Here's the drawing with two shaded views (mm, measured from the low corner). I have some questions. Give positions to 0.01 mm unless a question says otherwise; leave off trailing zeros. Order: outer loops, then holes, each group sorted by start corner. A loop starts at its lowest first (then second) coordinate and runs counter-clockwise, first axis right, second up. Notation, with made-up numbers: M 42.5,13 L 59.5,13 A6 cw 59.5,21 Z; hole C 7.5,87 d4. An arc over 180 degrees is marked long. Use a Markdown table: item, result. Add a question column.
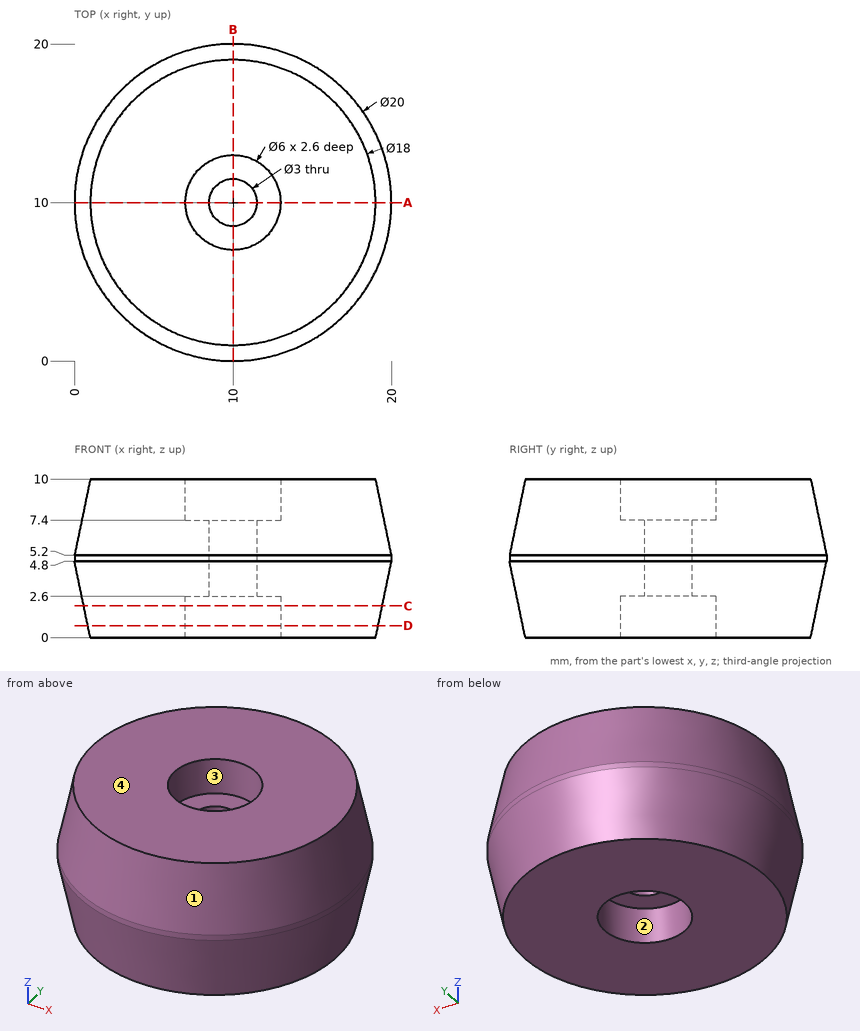
1) We'd pull the mould along X, two halves only. Please class the marked faces 1, 2, 3 and 4: pulls with the +X half, pulls with the -X half, needs draft (parallel to the pull), parting line crosses it, or undercut.
2) Suppose I cut it at D-D on z = 0.75. Please give me the cut outline in (x, y), and give its area (3 significant figures).
3) Please list where these lines run through material, in increasing order: line 1 (Y direction, x = 10.25, z = 1); line 2 (X direction, y = 11.75, z = 8.5); line 3 (Y direction, x = 8, z = 2.5). Write a range as from..to.
4) For pin 1 (5 mm diameter, centred on y = 14.5, z = 6.5, fed in from +X); pin 2 (3 mm diameter, centred on x = 6.5, z = 4, fed in from +Y); pin 3 (2.5 mm diameter, centred on x = 10, y = 10, fed in from +Z); pin 4 (1 mm diameter, centred on x = 14, z = 7.5, fed in from -Y), each with a flat end and sliding along its axis, tell me the tip position at first contact or that it passes through.
5) Suppose I cut it at A-A on y = 10. Please give me the cut outline in (x, z), and give its area (3 significant figures).
6) Suppose I cut it at C-C on z = 2. Please give me the cut outline in (x, y).
Values found:
| question | item | result |
|---|---|---|
| 1 | face 1 | parting line crosses it |
| 1 | face 2 | undercut |
| 1 | face 3 | undercut |
| 1 | face 4 | needs draft |
| 2 | outline | C 10,10 d18.31; hole C 10,10 d6 |
| 2 | area | 235 mm^2 |
| 3 | line 1 | y = 0.8..7.01, 12.99..19.2 |
| 3 | line 2 | x = 0.85..7.56, 12.44..19.15 |
| 3 | line 3 | y = 0.69..7.76, 12.24..19.31 |
| 4 | pin 1 | stops at x = 19.72 |
| 4 | pin 2 | stops at y = 19.75 |
| 4 | pin 3 | passes through |
| 4 | pin 4 | stops at y = 1.12 |
| 5 | outline | M 0,4.8 L 1,0 L 7,0 L 7,2.6 L 8.5,2.6 L 8.5,7.4 L 7,7.4 L 7,10 L 1,10 L 0,5.2 Z; M 11.5,2.6 L 13,2.6 L 13,0 L 19,0 L 20,4.8 L 20,5.2 L 19,10 L 13,10 L 13,7.4 L 11.5,7.4 Z |
| 5 | area | 145 mm^2 |
| 6 | outline | C 10,10 d18.83; hole C 10,10 d6 |
